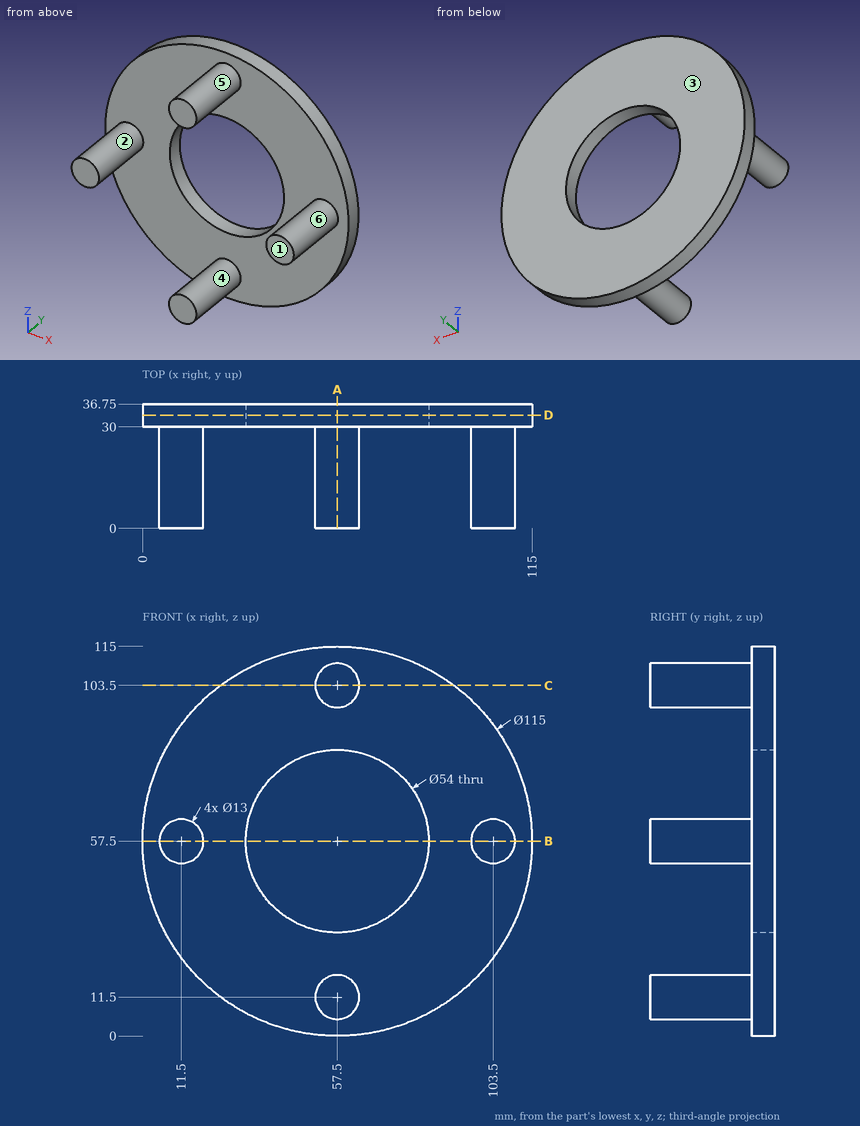
The figure shows three views and two pictorial views of one solid part (mm, origin at its lowest corner). Answer the questions. A direction names the side the tool comes from. Coordinates: 2 decimals unless noted, no trailing zeros. Loops run counter-clockwise (first coordinate to the right, second up) from the corner with the lowest first, then second, coordinate; pieces in that order, holes last. Notation, with made-up numbers: (66, -35.5) - (84, -35.5) arc R27 cw to (84, -2.5) - close; hole circle Ø11 at (53.25, 56). An arc over 180 degrees is marked (long way). Use a Markdown table: item, result. Add a question column.
1) The mould has two halves that part along Z. Classify the marked faces 3, 4, 5 and 6: released by +Z, released by -Z, zero draft, split by the parting line, or undercut.
2) The part is cut by section D-D, the plane y = 33.5. Give the vertices of the cut face in (x, z), and give its area (3 significant figures).
3) The part is cut by section B-B, the plane z = 57.5. Give the vertices of the cut face in (x, y), and give its area (3 significant figures).
4) The part is cut by section C-C, the plane z = 103.5. Give the vertices of the cut face in (x, y), and give its area (3 significant figures).
5) Find the intervals of material crossed by line 1 (X direction, y = 33.75, z = 57.5); line 2 (Y direction, x = 74, z = 29), in increasing order.
6) For the marked faces 1 and 2, determine the directions among +Z, -Z, +X, -X, +Y, -Y from which every point of the face is accessible in a straight line to the end or side of a thin tool.
7) Given pin 1 (12 mm diameter, centred on x = 58.5, y = 5.5, fed in from +Z); pin 2 (1.5 mm diameter, centred on x = 97, y = 19, fed in from +Z); pin 3 (3 mm diameter, centred on y = 14, z = 96.5, fed in from -X), each flat-ended and moving along its own axis, determine where each tip first touches the part or whether it passes through.
8) The part is cut by section A-A, the plane x = 57.5. Give the vertices of the cut face in (y, z).
Here are the results:
| question | item | result |
|---|---|---|
| 1 | face 3 | zero draft |
| 1 | face 4 | undercut |
| 1 | face 5 | undercut |
| 1 | face 6 | split by the parting line |
| 2 | outline | circle Ø115 at (57.5, 57.5); hole circle Ø54 at (57.5, 57.5) |
| 2 | area | 8,100 mm^2 |
| 3 | outline | (0, 30) - (5, 30) - (5, 0) - (18, 0) - (18, 30) - (30.5, 30) - (30.5, 36.75) - (0, 36.75) - close; (84.5, 30) - (97, 30) - (97, 0) - (110, 0) - (110, 30) - (115, 30) - (115, 36.75) - (84.5, 36.75) - close |
| 3 | area | 1,190 mm^2 |
| 4 | outline | (23, 30) - (51, 30) - (51, 0) - (64, 0) - (64, 30) - (92, 30) - (92, 36.75) - (23, 36.75) - close |
| 4 | area | 856 mm^2 |
| 5 | line 1 | x = 0 to 30.5, 84.5 to 115 |
| 5 | line 2 | y = 30 to 36.75 |
| 6 | face 1 | +Z, -Z, +X, -X, -Y |
| 6 | face 2 | -Y |
| 7 | pin 1 | stops at z = 110 |
| 7 | pin 2 | stops at z = 60.53 |
| 7 | pin 3 | stops at x = 54.04 |
| 8 | outline | (0, 5) - (30, 5) - (30, 0) - (36.75, 0) - (36.75, 30.5) - (30, 30.5) - (30, 18) - (0, 18) - close; (0, 97) - (30, 97) - (30, 84.5) - (36.75, 84.5) - (36.75, 115) - (30, 115) - (30, 110) - (0, 110) - close |
